CAD build for the part. Positions are in the model's coordinates, mm. A direction names the side the tool comes from. Coordinates: 2 decimals unless noted, no trailing zeros. Write each loop counter-clockwise with the first axis right and the second up, starting at its lowest first coordinate (ties: lowest second). Pieces come first, ordered by that corner, then holes. Notation, with made-up numbers: (75.5, 50.25) - (130.5, 50.25) arc R12 cw to (130.5, 64.25) - close; hole circle Ø7 at (19, -25). An arc over 180 degrees is marked (long way). Answer in a Markdown table with one row per item. Add a question column.
Q1. Two-plate mould, pull along X, no slides. Class faces 6 (the flat face through (3.86, 24.65, -9.11)), 7 (the flat face through (9.087, 24.65, -3.842)), 8 (the flat face through (-10, 25, -7)): +X half, -X half, draft (parallel to the pull), parting line (faces both ways), or undercut.
Q2. Band-saw the part on B-B (z = 0). List the corners of the cut face in (x, y), and give its area (3 significant figures).
Q3. Pin check, flat tips, straight feed: pin 1 (6 mm diameter, centred on x = -1, y = 41.5, fed in from -Z); pin 2 (10 mm diameter, centred on y = 33.5, z = 3.5, fed in from +X); pin 3 (1.5 mm diameter, centred on x = 1.5, z = -7.5, fed in from +Y); pin 4 (6 mm diameter, centred on y = 29, z = 0, fed in from -X). Stop position of each tip, or through.
Q4. Band-saw the part on A-A (x = 0). List the corners of the cut face in (y, z).
Q5. Drill centre lines: line 1 along Z through (x, y) = (0, 39); line 2 along Z through (x, y) = (5, 27). Where is each one in solid material? Low to high. Write a range as from..to.
Q6. 3-axis set-ups, long thin cutter, end or side, ignore diameter. For faces 1 (the flat face through (-4, 25, -8.2)), 2 (the flat face through (-3.842, 24.65, -9.087)), 3 (the flat face through (0, 25, 3.9)), 4 (the flat face through (-3.9, 25, 0)), 5 (the flat face through (3.9, 25, 0)): which of +Z, -Z, +X, -X, +Y, -Y reach the whole face in a straight line?
```python
from build123d import *

# Parameters (mm, degrees)
SKETCH1_R           = 2.1
BOSS_EXTRUDE1_DEPTH = 50


with BuildPart() as part:
    # Sketch1 → Boss-Extrude1 (new body)
    with BuildSketch(Plane(origin=(0, 0, 0), x_dir=(1, 0, 0), z_dir=(0, 1, 0))):
        with BuildLine():
            Line((-5.5, 8.2), (-3.125, 8.2))
            Line((-3.125, 8.2), (-4.58, 10))
            Line((-4.58, 10), (-9, 10))
            ThreePointArc((-9, 10), (-9.707106781, 9.707106781), (-10, 9))
            Line((-10, 9), (-10, 4.58))
            Line((-10, 4.58), (-8.2, 3.125))
            Line((-8.2, 3.125), (-8.2, 5.5))
            Line((-8.2, 5.5), (-6.56, 5.5))
            Line((-6.56, 5.5), (-3.9, 2.84))
            Line((-3.9, 2.84), (-3.9, -2.84))
            Line((-3.9, -2.84), (-6.56, -5.5))
            Line((-6.56, -5.5), (-8.2, -5.5))
            Line((-8.2, -5.5), (-8.2, -3.125))
            Line((-8.2, -3.125), (-10, -4.58))
            Line((-10, -4.58), (-10, -9))
            ThreePointArc((-10, -9), (-9.707106781, -9.707106781), (-9, -10))
            Line((-9, -10), (-4.58, -10))
            Line((-4.58, -10), (-3.125, -8.2))
            Line((-3.125, -8.2), (-5.5, -8.2))
            Line((-5.5, -8.2), (-5.5, -6.56))
            Line((-5.5, -6.56), (-2.84, -3.9))
            Line((-2.84, -3.9), (2.84, -3.9))
            Line((2.84, -3.9), (5.5, -6.56))
            Line((5.5, -6.56), (5.5, -8.2))
            Line((5.5, -8.2), (3.125, -8.2))
            Line((3.125, -8.2), (4.58, -10))
            Line((4.58, -10), (9, -10))
            ThreePointArc((9, -10), (9.707106781, -9.707106781), (10, -9))
            Line((10, -9), (10, -4.58))
            Line((10, -4.58), (8.2, -3.125))
            Line((8.2, -3.125), (8.2, -5.5))
            Line((8.2, -5.5), (6.56, -5.5))
            Line((6.56, -5.5), (3.9, -2.84))
            Line((3.9, -2.84), (3.9, 2.84))
            Line((3.9, 2.84), (6.56, 5.5))
            Line((6.56, 5.5), (8.2, 5.5))
            Line((8.2, 5.5), (8.2, 3.125))
            Line((8.2, 3.125), (10, 4.58))
            Line((10, 4.58), (10, 9))
            ThreePointArc((10, 9), (9.707106781, 9.707106781), (9, 10))
            Line((9, 10), (4.58, 10))
            Line((4.58, 10), (3.125, 8.2))
            Line((3.125, 8.2), (5.5, 8.2))
            Line((5.5, 8.2), (5.5, 6.56))
            Line((5.5, 6.56), (2.84, 3.9))
            Line((2.84, 3.9), (-2.84, 3.9))
            Line((-2.84, 3.9), (-5.5, 6.56))
            Line((-5.5, 6.56), (-5.5, 8.2))
        make_face()
        Circle(SKETCH1_R, mode=Mode.SUBTRACT)
    extrude(amount=BOSS_EXTRUDE1_DEPTH)


solid = part.part
```
Checked values:
| question | item | result |
|---|---|---|
| 1 | face 6 | undercut |
| 1 | face 7 | +X half |
| 1 | face 8 | -X half |
| 2 | outline | (-3.9, 0) - (-2.1, 0) - (-2.1, 50) - (-3.9, 50) - close; (2.1, 0) - (3.9, 0) - (3.9, 50) - (2.1, 50) - close |
| 2 | area | 180 mm² |
| 3 | pin 1 | stops at z = -9.28 |
| 3 | pin 2 | stops at x = 10 |
| 3 | pin 3 | passes through |
| 3 | pin 4 | stops at x = -4.06 |
| 4 | outline | (0, -3.9) - (50, -3.9) - (50, -2.1) - (0, -2.1) - close; (0, 2.1) - (50, 2.1) - (50, 3.9) - (0, 3.9) - close |
| 5 | line 1 | z = -3.9..-2.1, 2.1..3.9 |
| 5 | line 2 | z = -10..-8.2, -6.06..-3.94, 3.94..6.06, 8.2..10 |
| 6 | face 1 | +Y, -Y |
| 6 | face 2 | -Z, +Y, -Y |
| 6 | face 3 | +Z, +Y, -Y |
| 6 | face 4 | -X, +Y, -Y |
| 6 | face 5 | +X, +Y, -Y |
